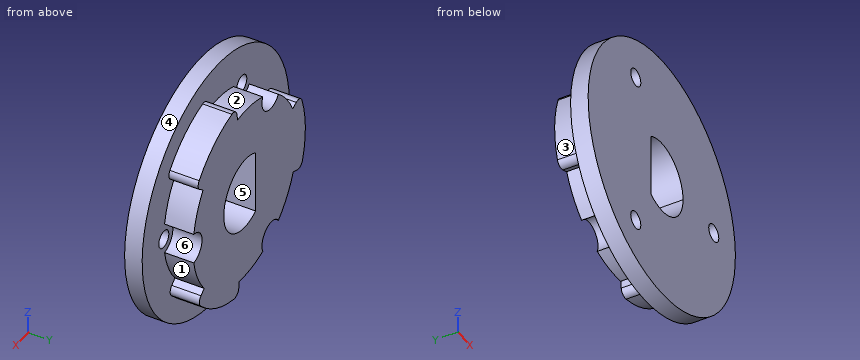
```python
from build123d import *

# Parameters (mm, degrees)
SKETCH1_R           = 19.54
SKETCH1_R_2         = 15.54
BOSS_EXTRUDE1_DEPTH = 7.9
SKETCH1_3_R         = 2.7
BOSS_EXTRUDE2_DEPTH = 7.9
SKETCH1_4_R         = 1.5
CUT_EXTRUDE1_DEPTH  = 29.740793308
CUT_EXTRUDE2_DEPTH  = 29.740793308
SKETCH1_6_R         = 1.5
CUT_EXTRUDE5_DEPTH  = 3
CIRPATTERN1_COUNT   = 3
SKETCH2_R           = 26
SKETCH2_R_2         = 19.54
BOSS_EXTRUDE3_DEPTH = 7.9
CUT_EXTRUDE4_START  = 7.9
SKETCH2_3_R         = 22
SKETCH2_3_R_2       = 19.54
CUT_EXTRUDE4_DEPTH  = 3.14
CUT_EXTRUDE6_START  = 3
SKETCH2_4_R         = 22
CUT_EXTRUDE6_DEPTH  = 3
BOSS_EXTRUDE5_DEPTH = 5
SKETCH5_R           = 22
BOSS_EXTRUDE6_DEPTH = 3
SKETCH6_R           = 1.5
CUT_EXTRUDE7_DEPTH  = 3
CUT_EXTRUDE8_DEPTH  = 15


with BuildPart() as part:
    # Sketch1 → Boss-Extrude1 (new body)
    with BuildSketch(Plane(origin=(0, 0, 0), x_dir=(1, 0, 0), z_dir=(0, 1, 0))):
        with Locations(Location((0, 0, 0), (0, 0, 270))):
            Circle(SKETCH1_R)
        with Locations(Location((0, 0, 0), (0, 0, 270))):
            Circle(SKETCH1_R_2, mode=Mode.SUBTRACT)
    extrude(amount=BOSS_EXTRUDE1_DEPTH)

    # Sketch1<3> → Boss-Extrude2 (add)
    with BuildSketch(Plane(origin=(0, 0, 0), x_dir=(1, 0, 0), z_dir=(0, 1, 0))):
        with Locations((15.54, 0)):
            Circle(SKETCH1_3_R)
    boss_extrude2 = extrude(amount=BOSS_EXTRUDE2_DEPTH)

    # Sketch1<4> → Cut-Extrude1 (cut, symmetric)
    with BuildSketch(Plane(origin=(0, 0, 0), x_dir=(1, 0, 0), z_dir=(0, 1, 0))):
        with Locations(Location((15.54, 0, 0), (0, 0, 270))):
            Circle(SKETCH1_4_R)
    cut_extrude1 = extrude(amount=CUT_EXTRUDE1_DEPTH, both=True, mode=Mode.SUBTRACT)

    # Sketch1<5> → Cut-Extrude2 (cut, symmetric)
    with BuildSketch(Plane(origin=(0, 0, 0), x_dir=(1, 0, 0), z_dir=(0, 1, 0))):
        with BuildLine():
            Line((1.84893352, 16.641004923), (1.716044464, 15.444960065))
            ThreePointArc((1.716044464, 15.444960065), (7.546281877, 13.584742538), (12.206193142, 9.617715372))
            Line((12.206193142, 9.617715372), (13.151430585, 10.362503249))
            ThreePointArc((13.151430585, 10.362503249), (13.623726964, 11.24345363), (13.299320972, 12.188915525))
            ThreePointArc((13.299320972, 12.188915525), (8.760291222, 15.770190161), (3.321432407, 17.731601359))
            ThreePointArc((3.321432407, 17.731601359), (2.347317501, 17.507463762), (1.84893352, 16.641004923))
        make_face()
    cut_extrude2 = extrude(amount=CUT_EXTRUDE2_DEPTH, both=True, mode=Mode.SUBTRACT)

    # Sketch1<6> → Cut-Extrude5 (cut)
    with BuildSketch(Plane(origin=(0, 0, 0), x_dir=(1, 0, 0), z_dir=(0, 1, 0))):
        with BuildLine():
            Line((13.541549805, -7.623518144), (14.590196156, -8.213877046))
            ThreePointArc((14.590196156, -8.213877046), (15.584628409, -8.315079224), (16.335293585, -7.655049543))
            ThreePointArc((16.335293585, -7.655049543), (17.48108114, -4.455715676), (18.006537967, -1.098267026))
            ThreePointArc((18.006537967, -1.098267026), (18.24, 0), (18.006537967, 1.098267026))
            ThreePointArc((18.006537967, 1.098267026), (17.48108114, 4.455715676), (16.335293585, 7.655049543))
            ThreePointArc((16.335293585, 7.655049543), (15.584628409, 8.315079224), (14.590196156, 8.213877046))
            Line((14.590196156, 8.213877046), (13.541549805, 7.623518144))
            ThreePointArc((13.541549805, 7.623518144), (14.632931196, 5.231531765), (15.305444015, 2.689792462))
            ThreePointArc((15.305444015, 2.689792462), (12.84, 0), (15.305444015, -2.689792462))
            ThreePointArc((15.305444015, -2.689792462), (14.632931196, -5.231531765), (13.541549805, -7.623518144))
        make_face()
        with Locations(Location((15.54, 0, 0), (0, 0, 270))):
            Circle(SKETCH1_6_R, mode=Mode.SUBTRACT)
    cut_extrude5 = extrude(amount=CUT_EXTRUDE5_DEPTH, mode=Mode.SUBTRACT)

    # CirPattern1: Boss-Extrude2, Cut-Extrude1, Cut-Extrude2, Cut-Extrude5 ×3 about axis
    cirpattern1_axis = Axis((0, 0, 0), (0, 1, 0))
    add([boss_extrude2.rotate(cirpattern1_axis, i * 360 / CIRPATTERN1_COUNT) for i in range(1, CIRPATTERN1_COUNT)])
    add([cut_extrude1.rotate(cirpattern1_axis, i * 360 / CIRPATTERN1_COUNT) for i in range(1, CIRPATTERN1_COUNT)], mode=Mode.SUBTRACT)
    add([cut_extrude2.rotate(cirpattern1_axis, i * 360 / CIRPATTERN1_COUNT) for i in range(1, CIRPATTERN1_COUNT)], mode=Mode.SUBTRACT)
    add([cut_extrude5.rotate(cirpattern1_axis, i * 360 / CIRPATTERN1_COUNT) for i in range(1, CIRPATTERN1_COUNT)], mode=Mode.SUBTRACT)

    # Sketch2 → Boss-Extrude3 (add)
    with BuildSketch(Plane(origin=(0, 0, 0), x_dir=(1, 0, 0), z_dir=(0, 1, 0))):
        with Locations(Location((0, 0, 0), (0, 0, 270))):
            Circle(SKETCH2_R)
        Circle(SKETCH2_R_2, mode=Mode.SUBTRACT)
    extrude(amount=BOSS_EXTRUDE3_DEPTH)

    # Sketch2<3> → Cut-Extrude4 (cut)
    with BuildSketch(Plane(origin=(0, 0, 0), x_dir=(1, 0, 0), z_dir=(0, 1, 0)).offset(CUT_EXTRUDE4_START)):
        with Locations(Location((0, 0, 0), (0, 0, 270))):
            Circle(SKETCH2_3_R)
        with Locations(Location((0, 0, 0), (0, 0, 270))):
            Circle(SKETCH2_3_R_2, mode=Mode.SUBTRACT)
    extrude(amount=-CUT_EXTRUDE4_DEPTH, mode=Mode.SUBTRACT)

    # Sketch2<4> → Cut-Extrude6 (cut)
    with BuildSketch(Plane(origin=(0, 0, 0), x_dir=(1, 0, 0), z_dir=(0, 1, 0)).offset(CUT_EXTRUDE6_START)):
        with Locations(Location((0, 0, 0), (0, 0, 270))):
            Circle(SKETCH2_4_R)
    extrude(amount=-CUT_EXTRUDE6_DEPTH, mode=Mode.SUBTRACT)


with BuildPart() as body_2:
    # Sketch4 → Boss-Extrude5 (new body)
    with BuildSketch(Plane(origin=(0, -20, 0), x_dir=(-1, 0, 0), z_dir=(0, -1, 0))):
        with BuildLine():
            Line((14.432282409, 5.762015659), (15.549906352, 6.208221358))
            ThreePointArc((15.549906352, 6.208221358), (16.548980018, 6.176766972), (17.205570975, 5.423092055))
            ThreePointArc((17.205570975, 5.423092055), (18.037530912, -0.298460376), (17.016733405, -5.989355912))
            ThreePointArc((17.016733405, -5.989355912), (16.335567089, -6.72089531), (15.335999768, -6.719279063))
            Line((15.335999768, -6.719279063), (14.233750009, -6.236341932))
            ThreePointArc((14.233750009, -6.236341932), (12.435838525, -9.318879771), (9.982150611, -11.910007102))
            ThreePointArc((9.982150611, -11.910007102), (6.42, -11.119766185), (5.323293404, -14.599799565))
            ThreePointArc((5.323293404, -14.599799565), (1.596947601, -15.457728111), (-2.226089267, -15.379731031))
            Line((-2.226089267, -15.379731031), (-2.398475768, -16.570724607))
            ThreePointArc((-2.398475768, -16.570724607), (-2.925252898, -17.420220588), (-3.906250001, -17.612007578))
            ThreePointArc((-3.906250001, -17.612007578), (-9.277239724, -15.471729803), (-13.695301074, -11.742245462))
            ThreePointArc((-13.695301074, -11.742245462), (-13.988249619, -10.786568429), (-13.487066248, -9.92172586))
            Line((-13.487066248, -9.92172586), (-12.517705544, -9.208618132))
            ThreePointArc((-12.517705544, -9.208618132), (-14.288305879, -6.110312195), (-15.305444015, -2.689792462))
            ThreePointArc((-15.305444015, -2.689792462), (-12.84, 0), (-15.305444015, 2.689792462))
            ThreePointArc((-15.305444015, 2.689792462), (-14.18525903, 6.345866865), (-12.206193142, 9.617715372))
            Line((-12.206193142, 9.617715372), (-13.151430585, 10.362503249))
            ThreePointArc((-13.151430585, 10.362503249), (-13.62372712, 11.243453616), (-13.299320974, 12.188915524))
            ThreePointArc((-13.299320974, 12.188915524), (-8.760291188, 15.770190179), (-3.32143233, 17.731601374))
            ThreePointArc((-3.32143233, 17.731601374), (-2.347317469, 17.507463739), (-1.84893352, 16.641004923))
            Line((-1.84893352, 16.641004923), (-1.716044464, 15.444960065))
            ThreePointArc((-1.716044464, 15.444960065), (1.852467354, 15.429191965), (5.323293404, 14.599799565))
            ThreePointArc((5.323293404, 14.599799565), (6.42, 11.119766185), (9.982150611, 11.910007102))
            ThreePointArc((9.982150611, 11.910007102), (12.588311429, 9.111861247), (14.432282409, 5.762015659))
        make_face()
    extrude(amount=BOSS_EXTRUDE5_DEPTH)

    # Sketch5 → Boss-Extrude6 (add)
    with BuildSketch(Plane.XZ.offset(25)):
        with Locations(Location((0, 0, 0), (0, 0, 270))):
            Circle(SKETCH5_R)
    extrude(amount=BOSS_EXTRUDE6_DEPTH)

    # Sketch6 → Cut-Extrude7 (cut)
    with BuildSketch(Plane(origin=(0, -25, 0), x_dir=(1, 0, 0), z_dir=(0, 1, 0))):
        with Locations(Location((-7.77, 13.458034775, 0), (0, 0, 270))):
            Circle(SKETCH6_R)
        with Locations(Location((15.54, 0, 0), (0, 0, 270))):
            Circle(SKETCH6_R)
        with Locations(Location((-7.77, -13.458034775, 0), (0, 0, 270))):
            Circle(SKETCH6_R)
    extrude(amount=-CUT_EXTRUDE7_DEPTH, mode=Mode.SUBTRACT)

    # Sketch7 → Cut-Extrude8 (cut)
    with BuildSketch(Plane.XZ.offset(28)):
        with BuildLine():
            ThreePointArc((6.35, 0), (3.175, 5.499261314), (-3.175, 5.499261314))
            Line((-3.175, 5.499261314), (-3.175, -5.499261314))
            ThreePointArc((-3.175, -5.499261314), (3.175, -5.499261314), (6.35, 0))
        make_face()
    extrude(amount=-CUT_EXTRUDE8_DEPTH, mode=Mode.SUBTRACT)


solid = body_2.part
```
Could you check a few things on this model? Use its own coordinates, in mm. Face numbers are marked on the shaded views. A direction names the side the tool comes from. Give positions to 0.01 mm unless a question says otherwise; leave off trailing zeros. Order: outer loops, then holes, each group sorted by start corner. A loop starts at its lowest first (then second) coordinate and runs counter-clockwise, first axis right, second up.
Q1. Suppose I cut it at D-D, the plane x = -7.77. Write out the boundary of the cut face in (y, z).
Q2. If I drill on line 1 along X through (y, z) = (-26.1, 0) (3 decimals); line 2 along Y through (x, z) = (-14.5, -10.5); line 3 along Z through (x, y) = (3.5, -20.5), over which ranges is the centre line in solid material (lowest first)?
Q3. I'm going to push flat-ended pins straight in: P1, Ø2.5, axis at x = 15.54, z = 0, coming from the -Y side; P2, Ø1, axis at x = 13.5, z = 17, coming from the +Y side; P3, Ø1.5, axis at y = -22.5, z = 3, coming from the +X side; P4, Ø2, axis at x = -17, y = -23.5, coming from the +Z side. Where does each tip first touch, or does it pass through?
Q4. Suppose I cut it at A-A, the plane x = 0. Write out the boundary of the cut face in (y, z).
Q5. For the marked faces 1, 2 and 3, which set-ups out of +Z, -Z, +X, -X, +Y, -Y let a thin tool reach every point of the face, with its end or its side?
Q6. Suppose I cut it at C-C, the plane y = -26.25. Write out the boundary of the cut face in (x, z) (3 decimals).
Q7. We'd pull the mould along X, two halves only. Please class the marked faces 4, 5 and 6: +X half, -X half, draft (parallel to the pull), parting line (faces both ways), or undercut.
Solution:
1. outline: (-28, -20.58) - (-25, -20.58) - (-25, -14.96) - (-28, -14.96) - close; (-28, -11.96) - (-25, -11.96) - (-25, -10.76) - (-20, -10.76) - (-20, 10.76) - (-25, 10.76) - (-25, 11.96) - (-28, 11.96) - close; (-28, 14.96) - (-25, 14.96) - (-25, 20.58) - (-28, 20.58) - close
2. line 1: x = -22 to -3.175, 6.35 to 14.04, 17.04 to 22
2. line 2: y = -28 to -25
2. line 3: z = -17.7 to -5.3, 5.3 to 17.63
3. P1: passes through
3. P2: stops at y = -25
3. P3: stops at x = 15.31
3. P4: stops at z = 6.81
4. outline: (-28, -22) - (-25, -22) - (-25, -15.54) - (-20, -15.54) - (-20, -6.35) - (-28, -6.35) - close; (-28, 6.35) - (-20, 6.35) - (-20, 15.54) - (-25, 15.54) - (-25, 22) - (-28, 22) - close
5. face 1: +X, +Y
5. face 2: +Z, +Y
5. face 3: -X, +Y
6. outline: circle Ø44 at (0, 0); hole circle Ø3 at (-7.77, -13.458); hole circle Ø3 at (-7.77, 13.458); hole (-3.175, -5.499) arc R6.35 ccw (long way) to (-3.175, 5.499) - close; hole circle Ø3 at (15.54, 0)
7. face 4: parting line
7. face 5: undercut
7. face 6: +X half
